from build123d import *

# Parameters (mm, degrees)
F2_W     = 1.8
F2_H     = 5.0446866744
F3_DEPTH = 12.5


with BuildPart() as f1:
    # F0 (on Front) → F1 (revolve)
    with BuildSketch(Plane.XZ):
        Polygon((-2.25, 0), (-1.5, 0), (-1.5, 7), (-3, 7), (-3, 6.5), (-2.25, 6.5), align=None)
    revolve(axis=Axis((0, 0, 1.9970234007), (0, 0, 1)))

    # F2 (on Front) → F3 (cut, symmetric)
    with BuildSketch(Plane.XZ):
        with Locations((0, 1.9776566628)):
            Rectangle(F2_W, F2_H)
    extrude(amount=F3_DEPTH, both=True, mode=Mode.SUBTRACT)


solid = f1.part
Geometry: final body of the model. Coordinates: model frame, mm. A direction names the side the tool comes from. Coordinates: 2 decimals unless noted, no trailing zeros. Order: outer loops, then holes, each group sorted by start corner. A loop starts at its lowest first (then second) coordinate and runs counter-clockwise, first axis right, second up.
(1) Material intervals for probe 1 along Y at (x, z) = (0, 4.75); probe 2 along X at (y, z) = (-0.65, 2.5), sorted ascending.
(2) Draft query along X for faces 1 (the face through (3, -0.1, 6.7)), 2 (the face through (-0.9, 1.6, 2.2)), 3 (the face through (-2, 0, 0)). Return one class per face: pulls with the +X half, pulls with the -X half, needs draft (parallel to the pull), parting line crosses it, or undercut.
(3) Section query C-C (z = 2.75). Return the cut outline in (x, y).
(4) Section query D-D (y = -1.8). Return the cut outline in (x, z).
(5) First-contact query: pin 1 (0.8 mm diameter, centred on x = 0, y = 2, fed in from -Z); pin 2 (1.8 mm diameter, centred on x = 0, y = 0, fed in from -Z); pin 3 (3 mm diameter, centred on x = -1.5, z = 2, fed in from -Y); pin 4 (0.7 mm diameter, centred on y = -1.5, z = 3.5, fed in from +X). Flat tips, straight axial feed; report the tip coordinate or a pass-through.
(6) Access query for faces 4 (the face through (-2.146, -0.676, 3.204)), 5 (the face through (0.9, 1.6, 2.2)), 6 (the face through (1.5, -0.07, 4.33)). Directions: +Z, -Z, +X, -X, +Y, -Y. A direction counts if a zero-diameter tool reaches every point of the face in a straight line with its end or side. Return the directions, or none.
(7) Section query A-A (x = 0). Return the cut outline in (y, z).
(8) Section query B-B (y = 0). Return the cut outline in (x, z), plus the area to 4 significant figures.
Solution:
1. probe 1: y = -2.25 to -1.5, 1.5 to 2.25
1. probe 2: x = -2.15 to -1.35, 1.35 to 2.15
2. face 1: parting line crosses it
2. face 2: undercut
2. face 3: needs draft
3. outline: (-0.9, -2.06) - (-0.9, -1.2) arc R1.5 cw to (-0.9, 1.2) - (-0.9, 2.06) arc R2.25 ccw to start; (0.9, -2.06) arc R2.25 ccw to (0.9, 2.06) - (0.9, 1.2) arc R1.5 cw to (0.9, -1.2) - close
4. outline: (-2.4, 6.5) - (-1.35, 6.5) - (-1.35, 0) - (-0.9, 0) - (-0.9, 4.5) - (0.9, 4.5) - (0.9, 0) - (1.35, 0) - (1.35, 6.5) - (2.4, 6.5) - (2.4, 7) - (-2.4, 7) - close
5. pin 1: stops at z = 4.5
5. pin 2: passes through
5. pin 3: stops at y = -2.06
5. pin 4: stops at x = 1.93
6. face 4: -Z
6. face 5: -Z, +Y, -Y
6. face 6: +Z, -Z
7. outline: (-3, 6.5) - (-2.25, 6.5) - (-2.25, 4.5) - (-1.5, 4.5) - (-1.5, 7) - (-3, 7) - close; (1.5, 4.5) - (2.25, 4.5) - (2.25, 6.5) - (3, 6.5) - (3, 7) - (1.5, 7) - close
8. outline: (-3, 6.5) - (-2.25, 6.5) - (-2.25, 0) - (-1.5, 0) - (-1.5, 7) - (-3, 7) - close; (1.5, 0) - (2.25, 0) - (2.25, 6.5) - (3, 6.5) - (3, 7) - (1.5, 7) - close
8. area: 11.25 mm2
